Here's how the part is built. I have some questions about the finished solid (model axes, mm). A direction names the side the tool comes from. Coordinates: 2 decimals unless noted, no trailing zeros. Loops run counter-clockwise (first coordinate to the right, second up) from the corner with the lowest first, then second, coordinate; pieces in that order, holes last. Notation, with made-up numbers: M -13.5,56.25 L 5.5,56.25 A26 cw 5.5,72.25 Z; hole C 44,5 d8. An arc over 180 degrees is marked long. Use one line per item in the form item = value. Start each with the question number.
(1) Imagine slicing it at C-C, the plane z = 39.5. Please give me the cut outline in (x, y).
(2) Please list where these lines run through material, in increasing order: L1, parallel to Z at x = 1, y = 9; L2, parallel to Z at x = 44, y = 8.5; L3, parallel to X at y = 2, z = 24.5.
(3) On a 3-axis mill with a long thin cutter (end or side, diameter ignored), from which of +Z, -Z, +X, -X, +Y, -Y can I reach the whole of each face in a straight line? I mean faces 1 (the cylindrical face through (12.999, 15.767, 39.386)), 2 (the flat face through (44, 10, 28)), 3 (the flat face through (-4, 10, 30.7)). Say none if no direction works.
(4) Will these pins go through, and if not, where does the flat tip stop? P1, Ø6, axis at y = 11, z = 35.5, coming from the +X side; P2, Ø8, axis at x = 44.5, y = 13, coming from the -Z side; P3, Ø2, axis at x = 43.5, y = 9, coming from the +Z side.
(5) Imagine slicing it at D-D, the plane y = 17.25. Please give me the cut outline in (x, z).
(6) Imagine slicing it at A-A, the plane x = 10. Please give me the cut outline in (y, z).
(7) Imagine slicing it at B-B, the plane y = 10. Please give me the cut outline in (x, z), and give its area (3 significant figures).
Autodesk Inventor part; units mm, degrees
ref_plane "YZ Plane" through (0, 0, 0) normal (1, 0, 0) x (0, 1, 0)
ref_plane "XZ Plane" through (0, 0, 0) normal (0, 1, 0) x (-1, 0, 0)
ref_plane "XY Plane" through (0, 0, 0) normal (0, 0, 1) x (1, 0, 0)
sketch "Boceto1" plane through (0, 0, 0) normal (0, 0, 1) x (1, 0, 0)
  line L0 (0, 0) -> (40, 0)
  line L1 (40, 0) -> (40, 20)
  line L2 (40, 20) -> (0, 20)
  line L3 (0, 20) -> (0, 0)
  dimension "d0" = 40
  dimension "d1" = 20
extrude "Extrusión1" add sketch "Boceto1" along normal blind 28
sketch "Boceto2" plane through (0, 0, 28) normal (0, 0, 1) x (1, 0, 0)
  line L0 (0, 0) -> (40, 0)
  line L1 (-7.5, 20) -> (47.5, 20)
  line L2 (47.5, 20) -> (47.5, 0)
  line L3 (47.5, 0) -> (-7.5, 0)
  line L4 (-7.5, 0) -> (-7.5, 20)
  point P0 (20, 0)
  point P1 (20, 0)
  dimension "d4" = 55
extrude "Extrusión2" add sketch "Boceto2" along normal blind 2.7
sketch "Boceto3" plane through (0, 0, 30.7) normal (0, 0, 1) x (1, 0, 0)
  line L0 (0, 0) -> (40, 0)
  line L1 (40, 0) -> (40, 20)
  line L2 (40, 20) -> (0, 20)
  line L3 (0, 20) -> (0, 0)
  dimension "d7" = 40
  dimension "d8" = 20
extrude "Extrusión3" add sketch "Boceto3" along normal blind 7.7
sketch "Boceto4" plane through (0, 0, 38.4) normal (0, 0, 1) x (1, 0, 0)
  line L0 (0, 20) -> (0, 0)
  circle A0 centre (10, 10) radius 6.5
  dimension "d11" = 13
  dimension "d12" = 10
extrude "Extrusión4" add sketch "Boceto4" along normal blind 2
sketch "Boceto5" plane through (10, 10, 40.4) normal (0, 0, 1) x (1, 0, 0)
  circle A0 centre (0, 0) radius 6.5
  circle A1 centre (0, 0) radius 2.75
  point P0 (-10, -10)
  dimension "d15" = 5.5
extrude "Extrusión5" add sketch "Boceto5" along normal blind 4 contours A1
properties part number "Servo2"
Answer:
q1.outline = C 10,10 d13
q2.L1 = 0 to 38.4
q2.L2 = 28 to 30.7
q2.L3 = 0 to 40
q3.face_1 = +Z
q3.face_2 = -Z, +X, +Y, -Y
q3.face_3 = +Z, -X, +Y, -Y
q4.P1 = 40
q4.P2 = 28
q4.P3 = 30.7
q5.outline = M -7.5,28 L 0,28 L 0,0 L 40,0 L 40,28 L 47.5,28 L 47.5,30.7 L 40,30.7 L 40,38.4 L 0,38.4 L 0,30.7 L -7.5,30.7 Z
q6.outline = M 0,0 L 20,0 L 20,38.4 L 16.5,38.4 L 16.5,40.4 L 12.75,40.4 L 12.75,44.4 L 7.25,44.4 L 7.25,40.4 L 3.5,40.4 L 3.5,38.4 L 0,38.4 Z
q7.outline = M -7.5,28 L 0,28 L 0,0 L 40,0 L 40,28 L 47.5,28 L 47.5,30.7 L 40,30.7 L 40,38.4 L 16.5,38.4 L 16.5,40.4 L 12.75,40.4 L 12.75,44.4 L 7.25,44.4 L 7.25,40.4 L 3.5,40.4 L 3.5,38.4 L 0,38.4 L 0,30.7 L -7.5,30.7 Z
q7.area = 1,620 mm²
